```python
from build123d import *

# Parameters (mm, degrees)
F1_DEPTH = 9
F3_DEPTH = 40
F5_DEPTH = 9
F7_SIZE2 = 30
F7_SIZE  = 30


with BuildPart() as f1:
    # F0 (on Top) → F1 (new body)
    with BuildSketch(Plane.XY):
        with BuildLine():
            Line((418.25, -724.4302502657), (548.25, -949.5968552496))
            ThreePointArc((548.25, -949.5968552496), (1096.5, 0), (548.25, 949.5968552496))
            Line((548.25, 949.5968552496), (418.25, 724.4302502657))
            ThreePointArc((418.25, 724.4302502657), (836.5, 0), (418.25, -724.4302502657))
        make_face()
    extrude(amount=F1_DEPTH)

    # F2 (on face) → F3 (join)
    with BuildSketch(Plane.XY.offset(9)):
        with BuildLine():
            Line((547.9764372578, -653.0528877589), (550.5475876965, -656.1170655314))
            ThreePointArc((550.5475876965, -656.1170655314), (856.5, 0), (550.5475876965, 656.1170655314))
            Line((550.5475876965, 656.1170655314), (547.9764372578, 653.0528877589))
            ThreePointArc((547.9764372578, 653.0528877589), (852.5, 0), (547.9764372578, -653.0528877589))
        make_face()
    extrude(amount=F3_DEPTH)

    # F4 (on face) → F5 (join)
    with BuildSketch(Plane.XY):
        with BuildLine():
            Line((358.25, -620.5072018116), (418.25, -724.4302502657))
            ThreePointArc((418.25, -724.4302502657), (517.2313730049, -657.4222058765), (605.651725766, -576.9906733013))
            Line((605.651725766, -576.9906733013), (488.1538105677, -545.5072018115))
            Line((488.1538105677, -545.5072018115), (358.25, -620.5072018116))
        make_face()
    extrude(amount=F5_DEPTH)

    # F6: F1 across plane


with BuildPart() as f1_1:
    add(f1.part)
    add(f1.part.mirror(Plane.XZ))

    # F7
    f7_edges = [f1_1.edges().sort_by_distance(p)[0] for p in [
        (549.262012, -654.584977, 49),
        (549.262012, 654.584977, 49),
    ]]
    chamfer(f7_edges, length=F7_SIZE, length2=F7_SIZE2)


solid = f1_1.part
```
Geometry: final body of the model. Coordinates: model frame, mm. A direction names the side the tool comes from. Coordinates: 2 decimals unless noted, no trailing zeros. Loops run counter-clockwise (first coordinate to the right, second up) from the corner with the lowest first, then second, coordinate; pieces in that order, holes last. Notation, with made-up numbers: (51, 22) -> (95, 22) arc R16 cw to (95, 37) -> close; hole circle Ø2 at (47, 66). An arc over 180 degrees is marked (long way). Use a Markdown table: item, result. Add a question column.
(1) Line query: line 1 along Z through (x, y) = (873, -113); line 2 along Y through (x, z) = (626, 40.5) (3 decimals); line 3 along Y through (x, z) = (777, 36). Output: solid intervals per line, ascending.
(2) Pin query (flat end, axial travel): pin 1 Ø12 at (x, y) = (541, -654.5) entering from +Z; pin 2 Ø10 at (y, z) = (153, 19) entering from +X; pin 3 Ø5 at (x, z) = (467, 10.5) entering from +Y. Return the tip coordinate at first contact, or that it passes through.
(3) Section query D-D, the plane z = 27.5. Return loops of the section in (x, y), plus the area to 3 significant figures.
(4) Section query A-A, the plane x = 741.5. Return loops of the section in (y, z).
(5) Access query for faces 1 (the flat face through (547.73, 561.47, 4.44)), 2 (the flat face through (424.111, -582.482, 4.437)), 3 (the flat face through (886, -13, 0)), 4 (the cylindrical face through (852.436, 10.415, 28.72)), 5 (the flat face through (886, -13, 9)). Directions: +Z, -Z, +X, -X, +Y, -Y. A direction counts if a zero-diameter tool reaches every point of the face in a straight line with its end or side. Return the directions, or none.
(6) Section query C-C, the plane x = 520. Return loops of the section in (y, z).
(7) Mould query, pull axis Y, two halves, no side actions, for faces 6 (the flat face through (424.111, 582.482, 4.437)), 7 (the flat face through (451.92, 782.75, 4.44)), 8 (the cylindrical face through (856.436, -10.464, 28.72)), 9 (the flat face through (547.73, -561.47, 4.44)). Classes: pulls with the +Y half, pulls with the -Y half, needs draft (parallel to the pull), parting line crosses it, or undercut.
(8) Section query B-B, the plane y = 179.5. Return loops of the section in (x, z), plus the area to 3 significant figures.
Answer:
| question | item | result |
|---|---|---|
| 1 | line 1 | z = 0 to 9 |
| 1 | line 2 | y = -584.565 to -578.688, 578.688 to 584.565 |
| 1 | line 3 | y = -360.37 to -350.75, 350.75 to 360.37 |
| 2 | pin 1 | stops at z = 9 |
| 2 | pin 2 | stops at x = 843.62 |
| 2 | pin 3 | stops at y = 812.33 |
| 3 | outline | (554.46, -647.56) -> (557.03, -650.62) arc R856.5 ccw to (557.03, 650.62) -> (554.46, 647.56) arc R852.5 cw to start |
| 3 | area | 5,900 mm^2 |
| 4 | outline | (-807.77, 0) -> (-387.18, 0) -> (-387.18, 9) -> (-420.64, 9) -> (-420.64, 49) -> (-428.68, 49) -> (-428.68, 9) -> (-807.77, 9) -> close; (387.18, 0) -> (807.77, 0) -> (807.77, 9) -> (428.68, 9) -> (428.68, 49) -> (420.64, 49) -> (420.64, 9) -> (387.18, 9) -> close |
| 5 | face 1 | +Z, -Z |
| 5 | face 2 | +Z, -Z, -X |
| 5 | face 3 | -Z, +X, -X, +Y, -Y |
| 5 | face 4 | +Z, -X |
| 5 | face 5 | +Z |
| 6 | outline | (-900.67, 0) -> (-554.04, 0) -> (-554.04, 9) -> (-900.67, 9) -> close; (554.04, 0) -> (900.67, 0) -> (900.67, 9) -> (554.04, 9) -> close |
| 7 | face 6 | undercut |
| 7 | face 7 | pulls with the +Y half |
| 7 | face 8 | parting line crosses it |
| 7 | face 9 | undercut |
| 8 | outline | (817.01, 0) -> (1081.71, 0) -> (1081.71, 9) -> (837.48, 9) -> (837.48, 49) -> (833.39, 49) -> (833.39, 9) -> (817.01, 9) -> close |
| 8 | area | 2,550 mm^2 |
